Geometry: final body of the model. Coordinates: model frame, mm. A direction names the side the tool comes from. Give positions to 0.01 mm unless a question says otherwise; leave off trailing zeros. Write each loop counter-clockwise with the first axis right and the second up, starting at its lowest first coordinate (ties: lowest second). Pieces come first, ordered by that corner, then holes. Notation, with made-up numbers: M -19.5,-21 L -3.5,-21 A23 ccw -3.5,15 Z; hole C -35.75,29 d3. An arc over 180 degrees is marked long. Answer as a JSON object with one key per item and string values.
Autodesk Inventor part; units mm, degrees
ref_plane "YZ Plane" through (0, 0, 0) normal (1, 0, 0) x (0, 1, 0)
ref_plane "XZ Plane" through (0, 0, 0) normal (0, 1, 0) x (-1, 0, 0)
ref_plane "XY Plane" through (0, 0, 0) normal (0, 0, 1) x (1, 0, 0)
sketch "Sketch1" plane through (0, 0, 0) normal (1, 0, 0) x (0, 1, 0)
  line L0 (75, 5) -> (-75, 5)
  line L1 (-75, 5) -> (-75, -5)
  line L2 (-75, -5) -> (75, -5)
  line L3 (75, -5) -> (75, 5)
  line L4 (75, 5) -> (-75, -5) construction
  line L5 (-75, 5) -> (75, -5) construction
  point P0 (0, 0)
  dimension "d0" = 150
  dimension "d1" = 10
extrude "Extrusion1" add sketch "Sketch1" along normal blind 20
sketch "Sketch2" plane through (0, 75, 5) normal (0, 1, 0) x (1, 0, 0)
  line L0 (16.05, -5) -> (3.95, -5)
  line L1 (3.95, -5) -> (3.95, 5)
  line L2 (3.95, 5) -> (16.05, 5)
  line L3 (16.05, 5) -> (16.05, -5)
  line L4 (0, 0) -> (20, 0)
  line L5 (16.05, -5) -> (3.95, 5) construction
  line L6 (3.95, -5) -> (16.05, 5) construction
  point P0 (0, 5)
  point P1 (10, 0)
  point P2 (3.95, 0)
  point P3 (16.05, 0)
  dimension "d4" = 12.1
extrude "Extrusion2" cut sketch "Sketch2" against normal blind 145 contours L4 L1 L2 L3
sketch "Sketch3" plane through (3.95, 75, 0) normal (0, 0, 1) x (1, 0, 0)
  circle A0 centre (6.05, -134.5) radius 1.5
  line L0 (0, -145) -> (0, 0)
  line L1 (12.1, -145) -> (0, -145)
  circle A1 centre (6.05, -122.5) radius 1.5
  circle A2 centre (6.05, -122.5) radius 2.75
  circle A3 centre (6.05, -134.5) radius 2.75
  line L2 (1.5875, -111.5) -> (10.0422, -111.5)
  circle A4 centre (6.05, -88.5) radius 1.5
  circle A5 centre (6.05, -100.5) radius 1.5
  circle A6 centre (6.05, -100.5) radius 2.75
  circle A7 centre (6.05, -88.5) radius 2.75
  point P0 (-3.95, -75)
  point P1 (6.05, -145)
  dimension "d7" = 3
  dimension "d8" = 6.05
  dimension "d9" = 10.5
  dimension "d10" = 3
  dimension "d11" = 12
  dimension "d12" = 5.5
  dimension "d13" = 5.5
  dimension "d34" = 11
extrude "Extrusion3" cut sketch "Sketch3" against normal blind 5 contours A0 | A1 | A4 | A5
extrude "Extrusion4" cut sketch "Sketch3" against normal blind 2
sketch "Sketch4" plane through (0, 75, 5) normal (0, 1, 0) x (1, 0, 0)
  line L0 (0, 0) -> (0, 10)
  line L1 (0, 0) -> (0, 10)
  line L2 (20, 0) -> (20, 10)
  line L3 (0, 10) -> (20, 10)
  line L4 (20, 10) -> (20, 0)
  line L5 (16.05, 5) -> (16.05, 0)
  line L6 (20, 0) -> (16.05, 0)
  line L7 (3.95, 5) -> (16.05, 5)
  line L8 (16.05, 0) -> (16.05, 5)
  line L9 (16.05, 5) -> (3.95, 5)
  line L10 (3.95, 0) -> (3.95, 5)
  line L11 (3.95, 5) -> (3.95, 0)
  line L12 (3.95, 0) -> (0, 0)
  point P0 (0, 5)
extrude "Extrusion5" add sketch "Sketch4" along normal blind 30
sketch "Sketch6" plane through (3.95, -70, 0) normal (0, 0, 1) x (1, 0, 0)
  circle A0 centre (6.05, 169) radius 1.5
  circle A1 centre (6.05, 159) radius 1.5
  line L0 (0, 175) -> (12.1, 175)
  circle A2 centre (6.05, 169) radius 2.75
  circle A3 centre (6.05, 159) radius 2.75
  point P0 (-3.95, 70)
  point P1 (6.05, 175)
  dimension "d24" = 3
  dimension "d25" = 3
  dimension "d26" = 6
  dimension "d27" = 10
  dimension "d28" = 5.5
  dimension "d29" = 5.5
extrude "Extrusion6" cut sketch "Sketch6" against normal blind 5 contours A0 | A1
extrude "Extrusion7" cut sketch "Sketch6" against normal blind 2 contours A1 | A2 | A3
properties part number "Tiang Lifter_3DPrint"
1) Set-up query: faces 1 (the cylindrical face through (10, -49, -3)), 2 (the flat face through (16.05, 16, 2)), 3 (the cylindrical face through (9.642, -44.773, -0.986)). Return all of +Z, -Z, +X, -X, +Y, -Y with unobstructed straight access to the full face (end or side cutting, diameter ignored); none if empty.
Geometry check:
{"face 1": "+Z, -Z", "face 2": "+Z, +Y", "face 3": "+Z"}
2) Contact query for flat-ended pins moving along their axis: P1, Ø7, axis at x = 10, y = -13.5, coming from the +Z side; P2, Ø3, axis at x = 11, y = 98.5, coming from the +Z side; P3, Ø1.8, axis at x = 10, y = -25.5, coming from the +Z side. Output: stop coordinate, or through.
Geometry check:
{"P1": "stops at z = 0", "P2": "stops at z = -2", "P3": "passes through"}
3) Line query: line 1 (X direction, y = -1, z = 4.5); line 2 (X direction, y = 99, z = -2.8); line 3 (Z direction, x = 4, y = 69.5). Output: solid intervals per line, ascending. Write a range as from..to.
Geometry check:
{"line 1": "x = 0..3.95, 16.05..20", "line 2": "x = 0..8.5, 11.5..20", "line 3": "z = -5..0"}
4) Pull-direction query (X, two-part tool) for faces 4 (the flat face through (11, -49, -2)), 5 (the flat face through (17, 14, 5)), 6 (the flat face through (11, -27, -2)), 7 (the flat face through (0, 14, 0)); classes: pulls with the +X half, pulls with the -X half, needs draft (parallel to the pull), parting line crosses it, or undercut.
Geometry check:
{"face 4": "undercut", "face 5": "needs draft", "face 6": "undercut", "face 7": "pulls with the -X half"}
5) Cut plane A-A on y = -25.5. Return loops of the section in (x, z), and give its area (4 significant figures).
Geometry check:
{"outline": "M 0,-5 L 8.5,-5 L 8.5,-2 L 7.25,-2 L 7.25,0 L 3.95,0 L 3.95,5 L 0,5 Z; M 11.5,-5 L 20,-5 L 20,5 L 16.05,5 L 16.05,0 L 12.75,0 L 12.75,-2 L 11.5,-2 Z", "area": "119.5 mm2"}
6) Cut plane C-C on y = 53.5. Return loops of the section in (x, z).
Geometry check:
{"outline": "M 0,-5 L 20,-5 L 20,5 L 16.05,5 L 16.05,0 L 3.95,0 L 3.95,5 L 0,5 Z"}
7) Cut plane B-B on x = 10. Give the number of separate pieces and of enclosed holes in the cut face, and give its area (3 significant figures).
Geometry check:
{"separate pieces": "7", "enclosed holes": "0", "area": "805 mm2"}
